For this review, use the dimensioned drawing (mm, ordinates from the lowest corner) and the shaded views. Give positions to 0.01 mm unless a question says otherwise; leave off trailing zeros. Loops run counter-clockwise (first coordinate to the right, second up) from the corner with the lowest first, then second, coordinate; pieces in that order, holes last. Notation, with made-up numbers: (-31.5, 24) - (14.5, 24) arc R28 ccw to (14.5, 55) - close; hole circle Ø9 at (59.25, 24.25). An arc over 180 degrees is marked (long way). Put each result on its own line as item: value.
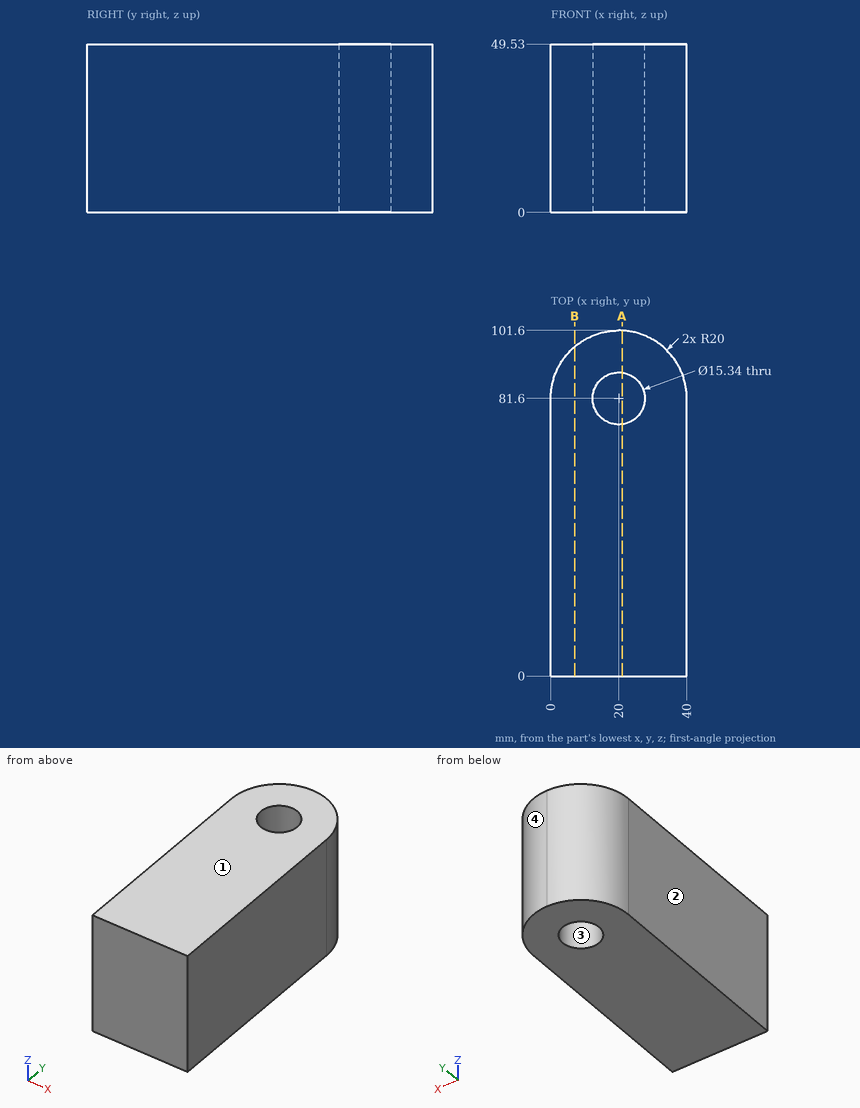
1) Insertion check: pin 1 Ø4 at (x, y) = (16, 70.5) entering from -Z; pin 2 Ø5 at (y, z) = (91, 34) entering from +X. Each pin has a flat end and moves straight along its axis. Give the tip position at first contact, or say it passes through.
Geometry check:
pin 1: stops at z = 0
pin 2: stops at x = 38.77
2) Wall thickness on line 1 (Y direction, x = 20, z = 34); line 2 (X direction, y = 81.6, z = 24); line 3 (X direction, y = 81, z = 16): over which ranges is each line inside the solid? List them lowest first.
Geometry check:
line 1: y = 0 to 73.93, 89.27 to 101.6
line 2: x = 0 to 12.33, 27.67 to 40
line 3: x = 0 to 12.35, 27.65 to 40
3) Take a section at B-B on x = 7. State the section outline as (y, z) points.
Geometry check:
outline: (0, 0) - (96.8, 0) - (96.8, 49.53) - (0, 49.53) - close
4) Take a section at A-A on x = 21. State the section outline as (y, z) points (1 decimal).
Geometry check:
outline: (0, 0) - (74, 0) - (74, 49.5) - (0, 49.5) - close; (89.2, 0) - (101.6, 0) - (101.6, 49.5) - (89.2, 49.5) - close
5) Draft analysis for pull direction X (two halves, no side actions). For the marked faces 1, 2, 3 and 4, state which applies: pulls with the +X half, pulls with the -X half, needs draft (parallel to the pull), parting line crosses it, or undercut.
Geometry check:
face 1: needs draft
face 2: pulls with the -X half
face 3: undercut
face 4: pulls with the +X half
